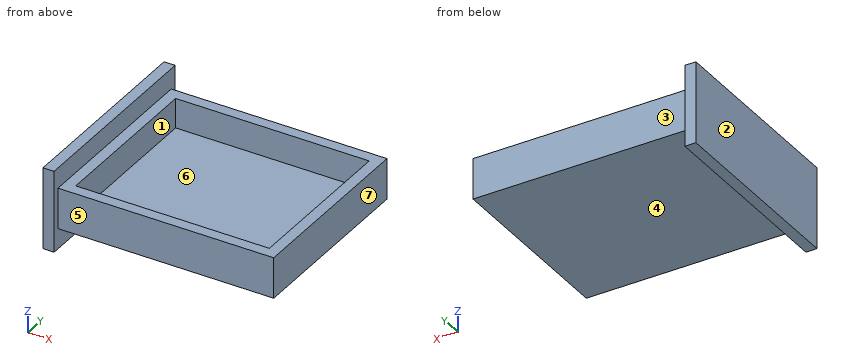
from build123d import *

# Parameters (mm, degrees)
F0_W     = 370
F0_H     = 320
F1_DEPTH = 70
F2_W     = 332
F2_H     = 282
F3_DEPTH = 51
F4_W     = 342
F4_H     = 140
F5_DEPTH = 19


with BuildPart() as f1:
    # F0 (on Top) → F1 (new body)
    with BuildSketch(Plane.XY):
        Rectangle(F0_W, F0_H)
    extrude(amount=F1_DEPTH)

    # F2 (on face) → F3 (cut)
    with BuildSketch(Plane.XY.offset(70)):
        Rectangle(F2_W, F2_H)
    extrude(amount=-F3_DEPTH, mode=Mode.SUBTRACT)

    # F4 (on face) → F5 (join)
    with BuildSketch(Plane(origin=(-185, 0, 0), x_dir=(0, -1, 0), z_dir=(-1, 0, 0))):
        with Locations((0, 35)):
            Rectangle(F4_W, F4_H)
    extrude(amount=F5_DEPTH)


solid = f1.part
Could you check a few things on this model? Use its own coordinates, in mm. Face numbers are marked on the shaded views. A direction names the side the tool comes from. Give positions to 0.01 mm unless a question says otherwise; leave off trailing zeros. Order: outer loops, then holes, each group sorted by start corner. A loop starts at its lowest first (then second) coordinate and runs counter-clockwise, first axis right, second up. Notation, with made-up numbers: (-7.5, 11.5) - (1.5, 11.5) arc R18 ccw to (1.5, 45.5) - close; hole circle Ø3 at (63.5, -23.75). An arc over 180 degrees is marked (long way). One line per question, with ' | ' between items. Start each with the question number.
Item 1: For the marked faces 1, 2, 3 and 4, which set-ups out of +Z, -Z, +X, -X, +Y, -Y let a thin tool reach every point of the face, with its end or its side?
Item 2: I'm going to push flat-ended pins straight in: pin 1 Ø8 at (x, y) = (-155, -24.5) entering from -Z; pin 2 Ø6 at (y, z) = (108.5, 88) entering from +X; pin 3 Ø8 at (x, z) = (77.5, 44) entering from +Y. Where does each tip first touch, or does it pass through?
Item 3: I want a section at A-A on z = 29. Write out the boundary of the cut face in (x, y), then the cut area to 3 significant figures.
Item 4: I want a section at C-C on x = -23.5. Write out the boundary of the cut face in (y, z), then the cut area to 3 significant figures.
Item 5: I want a section at D-D on z = -8. Write out the boundary of the cut face in (x, y).
Item 6: I want a section at B-B on y = 110.5. Write out the boundary of the cut face in (x, z), then the cut area to 3 significant figures.
Item 7: Thinking about a two-plate mould opening in X: for the marked faces 5, 6 and 7, which applies, pulls with the +X half, pulls with the -X half, needs draft (parallel to the pull), parting line crosses it, or undercut?
Item 8: I need wall thicknesses on probe 1 along X at (y, z) = (39, 23.5); probe 2 along Y at (x, z) = (58, 55.5); probe 3 along Z at (x, y) = (-6, -145.5). Which ranges of each line are inside material? Lowest first, please. Write a range as [from, to].
Verdict:
1) face 1: +Z | face 2: +Z, -Z, -X, +Y, -Y | face 3: +Z, -Z, +X, +Y | face 4: -Z, +X, +Y, -Y
2) pin 1: z = 0 | pin 2: x = -185 | pin 3: y = 160
3) outline: (-204, -171) - (-185, -171) - (-185, -160) - (185, -160) - (185, 160) - (-185, 160) - (-185, 171) - (-204, 171) - close; hole (-166, -141) - (166, -141) - (166, 141) - (-166, 141) - close | area: 31,300 mm^2
4) outline: (-160, 0) - (160, 0) - (160, 70) - (141, 70) - (141, 19) - (-141, 19) - (-141, 70) - (-160, 70) - close | area: 8,020 mm^2
5) outline: (-204, -171) - (-185, -171) - (-185, 171) - (-204, 171) - close
6) outline: (-204, -35) - (-185, -35) - (-185, 0) - (185, 0) - (185, 70) - (166, 70) - (166, 19) - (-166, 19) - (-166, 70) - (-185, 70) - (-185, 105) - (-204, 105) - close | area: 11,600 mm^2
7) face 5: needs draft | face 6: undercut | face 7: pulls with the +X half
8) probe 1: [-204, -166], [166, 185] | probe 2: [-160, -141], [141, 160] | probe 3: [0, 70]
